Check sheet for the modelled part. Datum: model origin and axes. Units: mm. Face numbers are marked on the shaded views. Give positions to 0.01 mm unless a question says otherwise; leave off trailing zeros. Loops run counter-clockwise (first coordinate to the right, second up) from the corner with the lowest first, then second, coordinate; pieces in that order, holes last. Notation, with made-up numbers: M -9,-1.75 L 43,-1.75 A22 ccw 43,37.25 Z; hole C 67,71 d2. An arc over 180 degrees is marked long. Use one line per item in the form item = value.
from build123d import *

# Parameters (mm, degrees)
BOSS_EXTRUDE1_DEPTH = 3


with BuildPart() as part:
    # Sketch1 → Boss-Extrude1 (new body)
    with BuildSketch(Plane(origin=(0, 0, 0), x_dir=(1, 0, 0), z_dir=(0, 1, 0))):
        with BuildLine():
            ThreePointArc((4.7625, 0), (0, -4.7625), (-4.7625, 0))
            Line((-4.7625, 0), (-4.7625, 8.248891971))
            ThreePointArc((-4.7625, 8.248891971), (-4.7625, -8.248891971), (9.525, 0))
            ThreePointArc((9.525, 0), (8.248891971, 4.7625), (4.7625, 8.248891971))
            Line((4.7625, 8.248891971), (4.7625, 0))
        make_face()
    extrude(amount=BOSS_EXTRUDE1_DEPTH)


solid = part.part
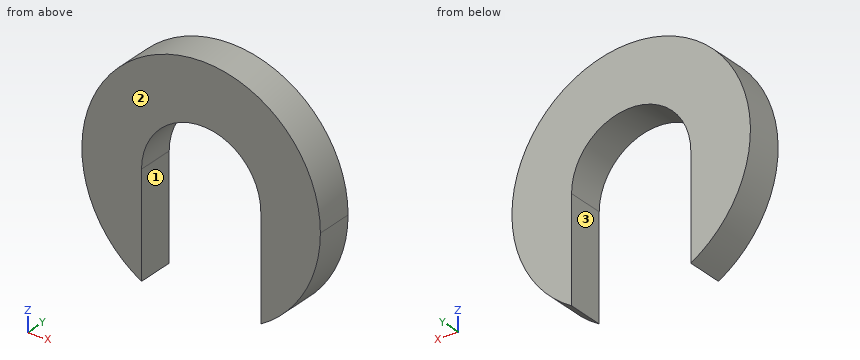
1) Section check A-A (z = -3.5). Record the cut outline in (x, y).
Evaluation:
outline = M -8.86,0 L -4.76,0 L -4.76,3 L -8.86,3 Z; M 4.76,0 L 8.86,0 L 8.86,3 L 4.76,3 Z
2) Section check C-C (z = 3). Record the cut outline in (x, y), then the cut area to 3 significant figures.
Evaluation:
outline = M -9.04,0 L -3.7,0 L -3.7,3 L -9.04,3 Z; M 3.7,0 L 9.04,0 L 9.04,3 L 3.7,3 Z
area = 32.0 mm^2
3) Section check D-D (x = 0). Record the cut outline in (y, z) (1 decimal), then the cut area to 3 significant figures.
Evaluation:
outline = M 0,4.8 L 3,4.8 L 3,9.5 L 0,9.5 Z
area = 14.3 mm^2
4) Scan lines: line 1 (X direction, y = 1.05, z = 3.75); line 2 (X direction, y = 0.4, z = -1.75); line 3 (Z direction, x = 6.75, y = 2.1). Record each from-to range of solid material in increasing order.
Evaluation:
line_1 = -8.76 to -2.94, 2.94 to 8.76
line_2 = -9.36 to -4.76, 4.76 to 9.36
line_3 = -6.72 to 6.72
5) Release check for a two-part mould opening along X. For the marked faces 1, 2 and 3 record: pulls with the +X half, pulls with the -X half, needs draft (parallel to the pull), parting line crosses it, or undercut.
Evaluation:
face_1 = undercut
face_2 = needs draft
face_3 = undercut
6) Depth check by flat-ended pin: pin 1 Ø8 at (x, z) = (1.5, -6.5) entering from -Y; pin 2 Ø1.5 at (y, z) = (2, -5) entering from +X; pin 3 Ø1 at (y, z) = (2.5, -1.5) entering from +X; pin 4 Ø1.5 at (x, y) = (2, 0.5) entering from -Z. Enter the tip coordinate at first touch or a pass-through.
Evaluation:
pin_1 = 0
pin_2 = 8.52
pin_3 = 9.47
pin_4 = 3.89
